Verification items for the finished model (mm, model axes). Coordinates: 2 decimals unless noted, no trailing zeros. Order: outer loops, then holes, each group sorted by start corner. A loop starts at its lowest first (then second) coordinate and runs counter-clockwise, first axis right, second up. Notation, with made-up numbers: (-2, 79) -> (34, 79) arc R24 ccw to (34, 100) -> close; hole circle Ø11 at (77, 50.5). An arc over 180 degrees is marked (long way). Write each question's results on one line, items separated by ' | '. Start each with the question number.
(1) Cross-section at A-A on y = 36.5. Enter the section's corners in (x, z).
(2) Go/stop test with flat-tipped pins: pin 1 (4 mm diameter, centred on x = 0, y = 36.5, fed in from +Z); pin 2 (3 mm diameter, centred on x = 24.5, y = 19, fed in from +Z). Record where each tip stops, or that it passes through.
(3) Thickness scan on probe 1 along Y at (x, z) = (-24.5, -30.4); probe 2 along Y at (x, z) = (0, -31.5). Record the ranges inside material, lowest first. Write a range as [from, to].
(4) Draft check along X on faces 1 (the cylindrical face through (-23.253, 18.483, -30.686)), 2 (the cylindrical face through (-27.1, 41.64, -30.69)), 3 (the cylindrical face through (27.14, 41.6, -30.69)). Enter one of: +X half, -X half, draft (parallel to the pull), parting line (faces both ways), or undercut.
(5) Cross-section at B-B on y = 19. Enter the section's corners in (x, z), and give its area (3 significant figures).
```python
from build123d import *

# Parameters (mm, degrees)
SKETCH010_R     = 1.35
PAD005_DEPTH    = 2
SKETCH011_R     = 1.5
POCKET003_DEPTH = 2.001
FILLET003_R     = 1


with BuildPart() as part:
    # Sketch010 → Pad005 (new body)
    with BuildSketch(Plane.XY):
        with BuildLine():
            Line((-28, 39.5), (-28, -39.5))
            ThreePointArc((-28, -39.5), (-27.12132, -41.62132), (-25, -42.5))
            Line((-25, -42.5), (25, -42.5))
            ThreePointArc((25, -42.5), (27.12132, -41.62132), (28, -39.5))
            Line((28, -39.5), (28, 39.5))
            ThreePointArc((28, 39.5), (27.12132, 41.62132), (25, 42.5))
            Line((25, 42.5), (-25, 42.5))
            ThreePointArc((-25, 42.5), (-27.12132, 41.62132), (-28, 39.5))
        make_face()
        with Locations((-24.5, 19)):
            Circle(SKETCH010_R, mode=Mode.SUBTRACT)
        with Locations((24.5, 19)):
            Circle(SKETCH010_R, mode=Mode.SUBTRACT)
        with Locations((24.5, -39)):
            Circle(SKETCH010_R, mode=Mode.SUBTRACT)
        with Locations((-24.5, -39)):
            Circle(SKETCH010_R, mode=Mode.SUBTRACT)
    extrude(amount=-PAD005_DEPTH)

    # Sketch011 (on Face13 of Pad005) → Pocket003 (cut, through all)
    with BuildSketch(Plane.XY):
        with Locations((0, 36.5)):
            Circle(SKETCH011_R)
        with Locations((0, -36.5)):
            Circle(SKETCH011_R)
    extrude(amount=-POCKET003_DEPTH, mode=Mode.SUBTRACT)

    # Fillet003
    fillet003_edges = [part.edges().sort_by_distance(p)[0] for p in [
        (-1.5, 36.5, 0),
        (-1.5, -36.5, 0),
    ]]
    fillet(fillet003_edges, radius=FILLET003_R)


with BuildPart() as part_1:
    # Body005 placement: moved
    add(part.part.moved(Location((0, 0, -29.7))))


solid = part_1.part
```
Results are:
1) outline: (-28, -31.7) -> (-1.5, -31.7) -> (-1.5, -30.7) arc R1 ccw to (-2.5, -29.7) -> (-28, -29.7) -> close; (1.5, -31.7) -> (28, -31.7) -> (28, -29.7) -> (2.5, -29.7) arc R1 ccw to (1.5, -30.7) -> close
2) pin 1: stops at z = -29.83 | pin 2: stops at z = -29.7
3) probe 1: y = [-42.5, -40.35], [-37.65, 17.65], [20.35, 42.5] | probe 2: y = [-42.5, -38], [-35, 35], [38, 42.5]
4) face 1: undercut | face 2: -X half | face 3: +X half
5) outline: (-28, -31.7) -> (-25.85, -31.7) -> (-25.85, -29.7) -> (-28, -29.7) -> close; (-23.15, -31.7) -> (23.15, -31.7) -> (23.15, -29.7) -> (-23.15, -29.7) -> close; (25.85, -31.7) -> (28, -31.7) -> (28, -29.7) -> (25.85, -29.7) -> close | area: 101 mm2
